from build123d import *

# Parameters (mm, degrees)
F0_W      = 116.327592
F0_H      = 88.219724
F1_DEPTH  = 48.768
F3_DEPTH  = 93.218
F5_DEPTH  = 21.082
F6_W      = 40.909464
F6_H      = 10.436087
F7_DEPTH  = 91.694
F8_W      = 33.952072
F8_H      = 17.108554
F9_DEPTH  = 78.486
F10_R     = 6.352216
F11_DEPTH = 58.928


with BuildPart() as f1:
    # F0 (on Top) → F1 (new body)
    with BuildSketch(Plane.XY):
        Rectangle(F0_W, F0_H)
    extrude(amount=F1_DEPTH)

    # F2 (on face) → F3 (cut)
    with BuildSketch(Plane.XZ.offset(44.109862)):
        Polygon((58.163796, 0), (58.163796, 48.768), (0, 48.768), align=None)
    extrude(amount=-F3_DEPTH, mode=Mode.SUBTRACT)

    # F4 (on face) → F5 (cut)
    with BuildSketch(Plane.XZ.offset(44.109862)):
        Polygon((58.163796, 0), (14.46391, 36.640594), (14.46391, 0), align=None)
    extrude(amount=-F5_DEPTH, mode=Mode.SUBTRACT)

    # F6 (on face) → F7 (cut)
    with BuildSketch(Plane.XZ.offset(44.109862)):
        with Locations((-37.709064, 5.218043)):
            Rectangle(F6_W, F6_H)
    extrude(amount=-F7_DEPTH, mode=Mode.SUBTRACT)

    # F8 (on face) → F9 (cut)
    with BuildSketch(Plane(origin=(-58.163796, 0, 0), x_dir=(0, -1, 0), z_dir=(-1, 0, 0))):
        with Locations((0, 48.768)):
            Rectangle(F8_W, F8_H)
    extrude(amount=-F9_DEPTH, mode=Mode.SUBTRACT)

    # F10 (on face) → F11 (cut)
    with BuildSketch(Plane(origin=(0, 0, 0), x_dir=(1, 0, 0), z_dir=(0, 0, -1))):
        with Locations((45.083895, 12.940748)):
            Circle(F10_R)
        with Locations((19.2024, 13.49734)):
            Circle(F10_R)
        with Locations((45.083895, -34.022748)):
            Circle(F10_R)
        with Locations((19.2024, -34.57934)):
            Circle(F10_R)
    extrude(amount=-F11_DEPTH, mode=Mode.SUBTRACT)


solid = f1.part
Part model, mm, in its own coordinate system. A direction names the side the tool comes from. Coordinates: 2 decimals unless noted, no trailing zeros. Write each loop counter-clockwise with the first axis right and the second up, starting at its lowest first coordinate (ties: lowest second). Pieces come first, ordered by that corner, then holes. Notation, with made-up numbers: (71, 69.25) - (85, 69.25) arc R23 ccw to (85, 96.25) - close; hole circle Ø7 at (38.5, -32). An arc over 180 degrees is marked (long way). Put each result on its own line as item: value.
1. Two-plate mould, pull along Y, no slides. Class faces 1 (the flat face through (-14, 44.11, 24)), 2 (the flat face through (-24, 16.976, 44)), 3 (the flat face through (26, -23.028, 10)), 4 (the flat face through (-29, -30, 48.768)): +Y half, -Y half, draft (parallel to the pull), parting line (faces both ways), or undercut.
Final values:
face 1: +Y half
face 2: undercut
face 3: -Y half
face 4: draft
2. Band-saw the part on B-B (y = 15.5). Write the cut outline in (x, z).
Final values:
outline: (-58.16, 10.44) - (-17.25, 10.44) - (-17.25, 0) - (58.16, 0) - (10.2, 40.21) - (-58.16, 40.21) - close
3. Flat gauge pins, fed straight in: pin 1 Ø23 at (y, z) = (-37.5, 25) entering from +X; pin 2 Ø14.5 at (x, y) = (19.2, 34.58) entering from +Z; pin 3 Ø1 at (y, z) = (-1.5, 34.5) entering from +X; pin 4 Ø11.5 at (y, z) = (6.5, 6) entering from -X. Where does each tip first touch, or does it go through?
Final values:
pin 1: stops at x = 14.46
pin 2: stops at z = 38.75
pin 3: stops at x = 17.61
pin 4: stops at x = -58.16
4. Band-saw the part on C-C (x = -49.5). Write the cut outline in (y, z), then the cut area to 3 significant figures.
Final values:
outline: (-44.11, 10.44) - (44.11, 10.44) - (44.11, 48.77) - (16.98, 48.77) - (16.98, 40.21) - (-16.98, 40.21) - (-16.98, 48.77) - (-44.11, 48.77) - close
area: 3,090 mm²
5. Band-saw the part on A-A (z = 23). Write the cut outline in (x, y).
Final values:
outline: (-58.16, -44.11) - (14.46, -44.11) - (14.46, -23.03) - (30.73, -23.03) - (30.73, 44.11) - (-58.16, 44.11) - close; hole circle Ø12.7 at (19.2, -13.5); hole circle Ø12.7 at (19.2, 34.58)
6. 3-axis set-ups, long thin cutter, end or side, ignore diameter. For faces 5 (the flat face through (-29, 31, 48.768)), 6 (the flat face through (14.464, -34, 19)), 7 (the flat face through (-17.254, -1, 5)), 8 (the flat face through (-24, 0, 40.214)), 9 (the cylindrical face through (38.738, -13.22, 6.306)): which of +Z, -Z, +X, -X, +Y, -Y reach the whole face in a straight line?
Final values:
face 5: +Z, +X, -X, +Y, -Y
face 6: +Z, -Z, +X, -Y
face 7: -Z, -X, +Y, -Y
face 8: +Z, +X, -X
face 9: +Z, -Z
7. Band-saw the part on D-D (z = 42.5). Write the cut outline in (x, y), then the cut area to 3 significant figures.
Final values:
outline: (-58.16, -44.11) - (7.48, -44.11) - (7.48, -16.98) - (-58.16, -16.98) - close; (-58.16, 16.98) - (7.48, 16.98) - (7.48, 44.11) - (-58.16, 44.11) - close
area: 3,560 mm²
8. Probe line 1 along X through (y, z) = (35, 5); line 2 along Y through (x, z) = (2, 42.5); line 3 along Z through (x, y) = (-52, 24). List the from-to ranges inside material, lowest first. Write a range as [from, to].
Final values:
line 1: x = [-17.25, 12.86], [25.54, 38.81], [51.36, 52.2]
line 2: y = [-44.11, -16.98], [16.98, 44.11]
line 3: z = [10.44, 48.77]
